Check sheet for the modelled part. Datum: model origin and axes. Units: mm. A direction names the side the tool comes from. Round coordinates to 2 decimals unless told otherwise and drop trailing zeros. Loops run counter-clockwise (first coordinate to the right, second up) from the corner with the lowest first, then second, coordinate; pieces in that order, holes last. Notation, with made-up numbers: (21.25, -33.5) -> (63.25, -33.5) arc R19 ccw to (63.25, -26.5) -> close; hole circle Ø10 at (74.5, 49). An arc over 180 degrees is marked (long way). One line per question, with ' | ' between items.
```python
from build123d import *

# Parameters (mm, degrees)
SKETCH_W         = 150
SKETCH_H         = 130
SKETCH_W_2       = 111
SKETCH_H_2       = 111
PAD_DEPTH        = 1.5
SKETCH001_W      = 150
SKETCH001_H      = 130
PAD001_DEPTH     = 8.5
HOLE_D           = 5
HOLE_DEPTH       = 25
HOLE_CSINK_D     = 10
HOLE_CSINK_ANGLE = 90


with BuildPart() as part:
    # Sketch → Pad (new body)
    with BuildSketch(Plane.XY):
        Rectangle(SKETCH_W, SKETCH_H)
        Rectangle(SKETCH_W_2, SKETCH_H_2, mode=Mode.SUBTRACT)
    extrude(amount=PAD_DEPTH)

    # Sketch001 (on Face10 of Pad) → Pad001 (join)
    with BuildSketch(Plane.XY.offset(1.5)):
        Rectangle(SKETCH001_W, SKETCH001_H)
    extrude(amount=PAD001_DEPTH)

    # Hole
    with Locations(Plane(origin=(0, 0, 0), x_dir=(1, 0, 0), z_dir=(0, 0, -1))):
        with Locations((-65, 55), (65, 55), (65, -55), (-65, -55)):
            CounterSinkHole(HOLE_D / 2, HOLE_CSINK_D / 2, depth=HOLE_DEPTH, counter_sink_angle=HOLE_CSINK_ANGLE)


solid = part.part
```
(1) Sectioned sample at B-B, the plane y = -22. Record the cut outline in (x, z), and give its area (3 significant figures).
Answer:
outline: (-75, 0) -> (-55.5, 0) -> (-55.5, 1.5) -> (55.5, 1.5) -> (55.5, 0) -> (75, 0) -> (75, 10) -> (-75, 10) -> close | area: 1,330 mm2
(2) Go/stop test with a flat-tipped pin: pin 1 (10 mm diameter, centred on x = 42, y = 33, fed in from -Z). Record where the tip stops, or that it passes through.
Answer:
pin 1: stops at z = 1.5
(3) Scan lines: probe 1 along Y at (x, z) = (65, 4.5); probe 2 along X at (y, z) = (-55, 7.5); probe 3 along Y at (x, z) = (-54.5, 1.25). Record each from-to range of solid material in increasing order.
Answer:
probe 1: y = -65 to -57.5, -52.5 to 52.5, 57.5 to 65 | probe 2: x = -75 to -67.5, -62.5 to 62.5, 67.5 to 75 | probe 3: y = -65 to -55.5, 55.5 to 65
(4) Sectioned sample at A-A, the plane x = 65. Record the cut outline in (y, z), and give its area (3 significant figures).
Answer:
outline: (-65, 0) -> (-60, 0) -> (-57.5, 2.5) -> (-57.5, 10) -> (-65, 10) -> close; (-52.5, 2.5) -> (-50, 0) -> (50, 0) -> (52.5, 2.5) -> (52.5, 10) -> (-52.5, 10) -> close; (57.5, 2.5) -> (60, 0) -> (65, 0) -> (65, 10) -> (57.5, 10) -> close | area: 1,190 mm2
(5) Set-up check for faces 4 (the face through (-1, 1, 10)), 5 (the face through (-1, 1, 1.5)): record each of +Z, -Z, +X, -X, +Y, -Y from which the full face is reachable in a straight line by a thin tool's end or side.
Answer:
face 4: +Z, +X, -X, +Y, -Y | face 5: -Z
(6) Sectioned sample at C-C, the plane x = 9.5. Record the cut outline in (y, z).
Answer:
outline: (-65, 0) -> (-55.5, 0) -> (-55.5, 1.5) -> (55.5, 1.5) -> (55.5, 0) -> (65, 0) -> (65, 10) -> (-65, 10) -> close
(7) Mould release check, pull along X, two halves, no side actions. Record for faces 1 (the face through (75, -1, 5)), 2 (the face through (-75, -1, 5)), 3 (the face through (-62.92, 56.595, 2.379)): +X half, -X half, draft (parallel to the pull), parting line (faces both ways), or undercut.
Answer:
face 1: +X half | face 2: -X half | face 3: undercut
